```python
from build123d import *

# Parameters (mm, degrees)
SKETCH3_R           = 2
CUT_EXTRUDE1_DEPTH  = 58.27924924
FILLET2_R           = 0.5
SKETCH4_R           = 18
SKETCH4_R_2         = 6
CUT_EXTRUDE2_DEPTH  = 6
CUT_EXTRUDE3_START  = -6
SKETCH5_R           = 18
CUT_EXTRUDE3_DEPTH  = 6
SKETCH6_R           = 10
BOSS_EXTRUDE1_DEPTH = 6
SKETCH8_R           = 8
BOSS_EXTRUDE2_DEPTH = 10
SKETCH10_R          = 6.5
CUT_EXTRUDE5_DEPTH  = 5
SKETCH11_R          = 10
BOSS_EXTRUDE3_DEPTH = 5
CUT_EXTRUDE6_START  = -5
SKETCH12_R          = 6.5
CUT_EXTRUDE6_DEPTH  = 5
SKETCH7_R           = 2.5
CUT_EXTRUDE8_DEPTH  = 58.279249356


with BuildPart() as part:
    # Sketch2 → Revolve1 (revolve)
    with BuildSketch(Plane.XY, mode=Mode.PRIVATE) as revolve1_sk:
        Polygon((-2.565200875, 0.515739462), (7.234799125, 0.515739462), (7.234799125, 5.515739462), (17.334799125, 5.515739462), (17.334799125, -18.484260538), (-12.665200875, -18.484260538), (-12.665200875, 5.515739462), (-2.565200875, 5.515739462), align=None)
    revolve(revolve1_sk.sketch.rotate(Axis((-12.665200875, -18.484260538, 0), (1, 0, 0)), 90), axis=Axis((-12.665200875, -18.484260538, 0), (1, 0, 0)))

    # Sketch3 → Cut-Extrude1 (cut, through all)
    with BuildSketch(Plane(origin=(17.334799125, 0, 0), x_dir=(0, 0, -1), z_dir=(1, 0, 0))):
        with Locations((0, -18.484260538)):
            Circle(SKETCH3_R)
    extrude(amount=-CUT_EXTRUDE1_DEPTH, mode=Mode.SUBTRACT)

    # Fillet2
    fillet2_edges = [part.edges().sort_by_distance(p)[0] for p in [
        (-2.565200875, -18.484260538, -24),
        (7.234799125, -18.484260538, -24),
        (17.334799125, -18.484260538, -24),
        (-12.665200875, -18.484260538, -24),
    ]]
    fillet(fillet2_edges, radius=FILLET2_R)

    # Sketch4 → Cut-Extrude2 (cut)
    with BuildSketch(Plane(origin=(17.334799125, 0, 0), x_dir=(0, 0, -1), z_dir=(1, 0, 0))):
        with Locations((0, -18.484260538)):
            Circle(SKETCH4_R)
        with Locations((0, -18.484260538)):
            Circle(SKETCH4_R_2, mode=Mode.SUBTRACT)
    extrude(amount=-CUT_EXTRUDE2_DEPTH, mode=Mode.SUBTRACT)

    # Sketch5 → Cut-Extrude3 (cut)
    with BuildSketch(Plane.ZY.offset(12.665200875).offset(CUT_EXTRUDE3_START)):
        with Locations(Location((0, -18.484260538, 0), (0, 0, 180))):
            Circle(SKETCH5_R)
    extrude(amount=CUT_EXTRUDE3_DEPTH, mode=Mode.SUBTRACT)

    # Sketch6 → Boss-Extrude1 (add, through all)
    with BuildSketch(Plane.ZY.offset(6.665200875)):
        with Locations((0, -18.484260538)):
            Circle(SKETCH6_R)
    extrude(amount=BOSS_EXTRUDE1_DEPTH)

    # Sketch8 → Boss-Extrude2 (add)
    with BuildSketch(Plane(origin=(17.334799125, 0, 0), x_dir=(0, 0, -1), z_dir=(1, 0, 0))):
        with Locations((0, -18.484260538)):
            Circle(SKETCH8_R)
    extrude(amount=-BOSS_EXTRUDE2_DEPTH)

    # Sketch10 → Cut-Extrude5 (cut)
    with BuildSketch(Plane.ZY.offset(12.665200875)):
        with Locations((0, -18.484260538)):
            Circle(SKETCH10_R)
    extrude(amount=-CUT_EXTRUDE5_DEPTH, mode=Mode.SUBTRACT)

    # Sketch11 → Boss-Extrude3 (add)
    with BuildSketch(Plane(origin=(17.334799125, 0, 0), x_dir=(0, 0, -1), z_dir=(1, 0, 0))):
        with Locations(Location((0, -18.484260538, 0), (0, 0, 180))):
            Circle(SKETCH11_R)
    extrude(amount=-BOSS_EXTRUDE3_DEPTH)

    # Sketch12 → Cut-Extrude6 (cut)
    with BuildSketch(Plane(origin=(17.334799125, 0, 0), x_dir=(0, 0, -1), z_dir=(1, 0, 0)).offset(CUT_EXTRUDE6_START)):
        with Locations(Location((0, -18.484260538, 0), (0, 0, 180))):
            Circle(SKETCH12_R)
    extrude(amount=CUT_EXTRUDE6_DEPTH, mode=Mode.SUBTRACT)

    # Sketch7 → Cut-Extrude8 (cut, through all)
    with BuildSketch(Plane.ZY.offset(12.665200875)):
        with Locations((0, -18.484260538)):
            Circle(SKETCH7_R)
    extrude(amount=-CUT_EXTRUDE8_DEPTH, mode=Mode.SUBTRACT)


solid = part.part
```
The model under review builds one solid part; all positions refer to its coordinate system, in mm. A direction names the side the tool comes from. Give positions to 0.01 mm unless a question says otherwise; leave off trailing zeros. Write each loop counter-clockwise with the first axis right and the second up, starting at its lowest first coordinate (ties: lowest second). Pieces come first, ordered by that corner, then holes.
(1) For P1, Ø10.5, axis at y = -16.5, z = 0.5, coming from the -X side; P2, Ø1.5, axis at x = -7, y = -31, coming from the -Z side; P3, Ø1.5, axis at y = -6, z = 4.5, coming from the +X side; P4, Ø11.5, axis at y = -18.48, z = 0, coming from the -X side, all flat-tipped, find the tip position at first contact; note any pin that passes through.
(2) Tool access review of faces 4 (the flat face through (12.335, -19, 3)), 5 (the flat face through (-6.665, -11, -8)), 6 (the flat face through (12.335, -27, 0)), 7 (the flat face through (-12.665, -18, 7)): name each direction out of +Z, -Z, +X, -X, +Y, -Y from which nothing blocks a thin tool from reaching the whole face with its end or side.
(3) The part is to be moulded in two halves that separate along Z. For faces 1 (the cylindrical face through (-7.55, 2.81, 11.07)), 2 (the flat face through (17.335, -1, -5)), 3 (the cylindrical face through (-9.62, -36.33, 2.34)), say which applies: released by +Z, released by -Z, zero draft, split by the parting line, or undercut.
(4) Consider section A-A, the plane x = -9.75. Give the boundary of the cut face in (y, z).
(5) Consider section B-B, the plane x = 10. Give the boundary of the cut face in (y, z).
(6) Consider section C-C, the plane x = 6.5. Give the boundary of the cut face in (y, z), and give its area (3 significant figures).
(7) To check wall thickness, follow L1, parallel to Y at x = 15.7, z = 0; L2, parallel to Y at x = 0.25, z = 0; L3, parallel to Z at x = 15.75, y = -20.5. State the ranges of each line that lie inside material, in increasing order.
Returned:
1. P1: stops at x = -12.67
1. P2: stops at z = -20.92
1. P3: stops at x = 11.33
1. P4: stops at x = -7.67
2. face 4: +X
2. face 5: -X
2. face 6: none
2. face 7: +Z, -Z, -X, +Y, -Y
3. face 1: split by the parting line
3. face 2: zero draft
3. face 3: undercut
4. outline: circle Ø48 at (-18.48, 0); circle Ø20 at (-18.48, 0); hole circle Ø36 at (-18.48, 0); hole circle Ø13 at (-18.48, 0)
5. outline: circle Ø48 at (-18.48, 0); hole circle Ø5 at (-18.48, 0)
6. outline: circle Ø38 at (-18.48, 0); hole circle Ø5 at (-18.48, 0)
6. area: 1,110 mm2
7. L1: y = -42.48 to -36.48, -28.48 to -24.98, -11.98 to -8.48, -0.48 to 5.52
7. L2: y = -37.48 to -20.98, -15.98 to 0.52
7. L3: z = -23.92 to -17.89, -9.79 to -6.18, 6.18 to 9.79, 17.89 to 23.92
